Autodesk Inventor part; units mm, degrees
ref_plane "YZ Plane" through (0, 0, 0) normal (1, 0, 0) x (0, 1, 0)
ref_plane "XZ Plane" through (0, 0, 0) normal (0, 1, 0) x (-1, 0, 0)
ref_plane "XY Plane" through (0, 0, 0) normal (0, 0, 1) x (1, 0, 0)
sketch "Sketch1" plane through (0, 0, 0) normal (0, 1, 0) x (-1, 0, 0)
  line L0 (0, 0) -> (-50, 0)
  line L1 (-50, -50) -> (0, -50)
  line L2 (-50, -41) -> (-47, -41)
  line L3 (-47, -41) -> (-47, -35)
  line L4 (-47, -35) -> (-50, -35)
  line L5 (-50, -35) -> (-50, -41) construction
  line L6 (-50, -9) -> (-47, -9)
  line L7 (-47, -9) -> (-47, -15)
  line L8 (-47, -15) -> (-50, -15)
  line L9 (-50, -15) -> (-50, -9) construction
  line L10 (-25, 0) -> (-25, -50) construction
  line L11 (-50, -9) -> (-50, 0)
  line L12 (-50, -15) -> (-50, -19)
  line L13 (-50, -41) -> (-50, -50)
  circle A0 centre (-47.75, -4) radius 1.25
  circle A1 centre (-47.75, -46) radius 1.25
  line L14 (-50, -31) -> (-42, -31)
  line L15 (-35, -31) -> (-35, -28.5)
  line L16 (-35, -28.5) -> (-39.7, -28.5)
  line L17 (-50, -19) -> (-42, -19)
  line L18 (-35, -19) -> (-35, -21.5)
  line L19 (-35, -21.5) -> (-39.7, -21.5)
  line L20 (-50, -31) -> (-50, -35)
  line L21 (-50, -28.5) -> (-50, -31) construction
  line L22 (-50, -21.5) -> (-50, -28.5)
  line L23 (-50, -19) -> (-50, -21.5) construction
  line L24 (-42, -32.35) -> (-39.7, -32.35)
  line L25 (-39.7, -32.35) -> (-39.7, -31)
  line L26 (-39.7, -27.15) -> (-42, -27.15)
  line L27 (-42, -27.15) -> (-42, -28.5)
  line L28 (-42, -31) -> (-42, -32.35)
  line L29 (-42, -28.5) -> (-42, -31) construction
  line L30 (-42, -22.85) -> (-39.7, -22.85)
  line L31 (-39.7, -22.85) -> (-39.7, -21.5)
  line L32 (-39.7, -17.65) -> (-42, -17.65)
  line L33 (-42, -17.65) -> (-42, -19)
  line L34 (-42, -21.5) -> (-42, -22.85)
  line L35 (-42, -19) -> (-42, -21.5) construction
  line L36 (-39.7, -28.5) -> (-39.7, -27.15)
  line L37 (-39.7, -31) -> (-39.7, -28.5) construction
  line L38 (-39.7, -21.5) -> (-39.7, -19) construction
  line L39 (-39.7, -19) -> (-39.7, -17.65)
  line L40 (-42, -31) -> (-39.7, -31) construction
  line L41 (-39.7, -31) -> (-35, -31)
  line L42 (-42, -28.5) -> (-50, -28.5)
  line L43 (-39.7, -28.5) -> (-42, -28.5) construction
  line L44 (-42, -21.5) -> (-50, -21.5)
  line L45 (-39.7, -21.5) -> (-42, -21.5) construction
  line L46 (-42, -19) -> (-39.7, -19) construction
  line L47 (-39.7, -19) -> (-35, -19)
  line L48 (0, -41) -> (-3, -41)
  line L49 (-3, -41) -> (-3, -35)
  line L50 (-3, -35) -> (0, -35)
  line L51 (0, -35) -> (0, -41) construction
  line L52 (0, -9) -> (-3, -9)
  line L53 (-3, -9) -> (-3, -15)
  line L54 (-3, -15) -> (0, -15)
  line L55 (0, -15) -> (0, -9) construction
  line L56 (0, -9) -> (0, 0)
  line L57 (0, -15) -> (0, -19)
  line L58 (0, -41) -> (0, -50)
  circle A2 centre (-2.25, -4) radius 1.25
  circle A3 centre (-2.25, -46) radius 1.25
  line L59 (0, -31) -> (-8, -31)
  line L60 (-15, -31) -> (-15, -28.5)
  line L61 (-15, -28.5) -> (-10.3, -28.5)
  line L62 (0, -19) -> (-8, -19)
  line L63 (-15, -19) -> (-15, -21.5)
  line L64 (-15, -21.5) -> (-10.3, -21.5)
  line L65 (0, -31) -> (0, -35)
  line L66 (0, -28.5) -> (0, -31) construction
  line L67 (0, -21.5) -> (0, -28.5)
  line L68 (0, -19) -> (0, -21.5) construction
  line L69 (-8, -32.35) -> (-10.3, -32.35)
  line L70 (-10.3, -32.35) -> (-10.3, -31)
  line L71 (-10.3, -27.15) -> (-8, -27.15)
  line L72 (-8, -27.15) -> (-8, -28.5)
  line L73 (-8, -31) -> (-8, -32.35)
  line L74 (-8, -28.5) -> (-8, -31) construction
  line L75 (-8, -22.85) -> (-10.3, -22.85)
  line L76 (-10.3, -22.85) -> (-10.3, -21.5)
  line L77 (-10.3, -17.65) -> (-8, -17.65)
  line L78 (-8, -17.65) -> (-8, -19)
  line L79 (-8, -21.5) -> (-8, -22.85)
  line L80 (-8, -19) -> (-8, -21.5) construction
  line L81 (-10.3, -28.5) -> (-10.3, -27.15)
  line L82 (-10.3, -31) -> (-10.3, -28.5) construction
  line L83 (-10.3, -21.5) -> (-10.3, -19) construction
  line L84 (-10.3, -19) -> (-10.3, -17.65)
  line L85 (-8, -31) -> (-10.3, -31) construction
  line L86 (-10.3, -31) -> (-15, -31)
  line L87 (-8, -28.5) -> (0, -28.5)
  line L88 (-10.3, -28.5) -> (-8, -28.5) construction
  line L89 (-8, -21.5) -> (0, -21.5)
  line L90 (-10.3, -21.5) -> (-8, -21.5) construction
  line L91 (-8, -19) -> (-10.3, -19) construction
  line L92 (-10.3, -19) -> (-15, -19)
  dimension "d0" = 50
  dimension "d1" = 50
  dimension "d20" = 3
  dimension "d21" = 6
  dimension "d22" = 6
  dimension "d26" = 20
  dimension "d27" = 2.5
  dimension "d28" = 2.25
  dimension "d30" = 2.5
  dimension "d31" = 2.25
  dimension "d32" = 5
  dimension "d33" = 15
  dimension "d34" = 2.5
  dimension "d35" = 15
  dimension "d36" = 2.5
  dimension "d37" = 4
  dimension "d38" = 5.2
  dimension "d39" = 2.3
  dimension "d40" = 8
  dimension "d41" = 2.3
  dimension "d42" = 5.2
  dimension "d43" = 8
  dimension "d44" = 5
extrude "Extrusion2" add sketch "Sketch1" along normal blind 6
equation "\"d22\" = d21"
equation "\"d30\" = d27"
equation "\"d31\" = d28"
equation "\"d33\" = d35"
equation "\"d34\" = d27"
equation "\"d36\" = d27"
equation "\"d43\" = d40"
properties part number "wall-front"
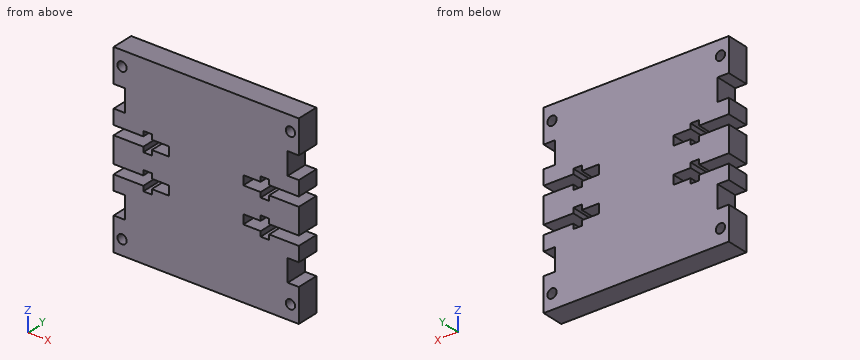
Model file for the job. Use its own axes, mm. Give positions to 0.01 mm unless a question says otherwise; leave off trailing zeros. Loops run counter-clockwise (first coordinate to the right, second up) from the corner with the lowest first, then second, coordinate; pieces in that order, holes last. Notation, with made-up numbers: (65.25, 73) - (77.25, 73) arc R23 cw to (77.25, 86) - close; hole circle Ø9 at (-30, -28.75). An arc over 180 degrees is marked (long way). One line per item, written item: value. Start each with the question number.
1. Pin check, flat tip, straight feed: pin 1 (1 mm diameter, centred on x = 43, z = -10.5, fed in from -Y). Stop position of the tip, or through.
2. Probe L1, parallel to X at y = 1.05, z = -22.5; L2, parallel to Z at x = 10, y = 5.65; L3, parallel to Z at x = 36, y = 4.5. List the from-to ranges inside material, lowest first. Write a range as from..to.
3. Slice it at A-A (x = 47.75). List the corners of the cut face in (y, z).
4. Slice it at C-C (y = 3.2). Give the number of separate pieces and of enclosed holes in the cut face, plus the area to 3 significant figures.
5. Slice it at B-B (z = -4). List the corners of the cut face in (x, y), plus the area to 3 significant figures.
Solution:
1. pin 1: stops at y = 0
2. L1: x = 0..8, 10.3..39.7, 42..50
2. L2: z = -50..-32.35, -27.15..-22.85, -17.65..0
2. L3: z = -50..-31, -28.5..-21.5, -19..0
3. outline: (0, -50) - (6, -50) - (6, -47.25) - (0, -47.25) - close; (0, -44.75) - (6, -44.75) - (6, -41) - (0, -41) - close; (0, -35) - (6, -35) - (6, -31) - (0, -31) - close; (0, -28.5) - (6, -28.5) - (6, -21.5) - (0, -21.5) - close; (0, -19) - (6, -19) - (6, -15) - (0, -15) - close; (0, -9) - (6, -9) - (6, -5.25) - (0, -5.25) - close; (0, -2.75) - (6, -2.75) - (6, 0) - (0, 0) - close
4. separate pieces: 1
4. enclosed holes: 4
4. area: 2,230 mm^2
5. outline: (0, 0) - (1, 0) - (1, 6) - (0, 6) - close; (3.5, 0) - (46.5, 0) - (46.5, 6) - (3.5, 6) - close; (49, 0) - (50, 0) - (50, 6) - (49, 6) - close
5. area: 270 mm^2
